```python
from build123d import *

# Parameters (mm, degrees)
F1_DEPTH = 12.7


with BuildPart() as f1:
    # F0 (on Top) → F1 (new body)
    with BuildSketch(Plane.XY):
        Polygon((-6.950833, -2.485712), (-10.236463, 1.818153), (-14.623778, -1.531184), (-11.338149, -5.835049), align=None)
        Polygon((-14.623778, -1.531184), (-10.236463, 1.818153), (-9.502501, 7.288792), (-12.851838, 11.676108), (-18.322477, 12.410069), (-22.709792, 9.060732), (-23.443754, 3.590093), (-20.094417, -0.797222), align=None)
    extrude(amount=F1_DEPTH)


solid = f1.part
```
Can you work these out from the model? Positions are in its coordinate system, mm. A direction names the side the tool comes from. Coordinates: 2 decimals unless noted, no trailing zeros. Loops run counter-clockwise (first coordinate to the right, second up) from the corner with the lowest first, then second, coordinate; pieces in that order, holes last. Notation, with made-up numbers: (-20.75, 57.25) -> (37.25, 57.25) arc R11 ccw to (37.25, 65.25) -> close; hole circle Ø11 at (-2.75, 18). An arc over 180 degrees is marked (long way). Put each result on its own line as item: value. Start each with the question number.
Q1. I'm going to push flat-ended pins straight in: P1, Ø5, axis at x = -14.5, z = 5.5, coming from the +Y side; P2, Ø4, axis at y = -2.5, z = 2.5, coming from the -X side; P3, Ø1, axis at x = -12, y = -2.5, coming from the -Z side. Where does each tip first touch, or does it pass through?
Q2. If I drill on line 1 (Y direction, x = -20.75, z = 2.25); line 2 (Y direction, x = -13.5, z = 8.25); line 3 (X direction, y = 1.5, z = 9), over which ranges is the centre line in solid material (lowest first)? Write a range as [from, to].
Q3. For faces 1 (the face through (-9.875, 4.515, 6.261)), 2 (the face through (-21.793, 1.427, 6.261)), which set-ups out of +Z, -Z, +X, -X, +Y, -Y let a thin tool reach every point of the face, with its end or its side?
Q4. Thinking about a two-plate mould opening in Y: for faces 3 (the face through (-17.4, -1.16, 6.26)), 4 (the face through (-8.571, -0.364, 6.261)), 5 (the face through (-15, 3, 0)), which applies, pulls with the +Y half, pulls with the -Y half, needs draft (parallel to the pull), parting line crosses it, or undercut?
Q5. I want a section at C-C (x = -19.75). Write out the boundary of the cut face in (y, z), plus the area to 3 significant figures.
Q6. I want a section at B-B (y = 5.5). Write out the boundary of the cut face in (x, z), plus the area to 3 significant figures.
Q7. I want a section at A-A (z = 8.75). Write out the boundary of the cut face in (x, y), plus the area to 3 significant figures.
Taken from the geometry:
1. P1: stops at y = 12.23
1. P2: stops at x = -20.32
1. P3: stops at z = 0
2. line 1: y = [0.06, 10.56]
2. line 2: y = [-3, 11.76]
2. line 3: x = [-21.85, -9.99]
3. face 1: +Z, -Z, +X
3. face 2: +Z, -Z, -X, -Y
4. face 3: pulls with the -Y half
4. face 4: undercut
4. face 5: needs draft
5. outline: (-0.84, 0) -> (11.32, 0) -> (11.32, 12.7) -> (-0.84, 12.7) -> close
5. area: 154 mm2
6. outline: (-23.19, 0) -> (-9.74, 0) -> (-9.74, 12.7) -> (-23.19, 12.7) -> close
6. area: 171 mm2
7. outline: (-23.44, 3.59) -> (-20.09, -0.8) -> (-14.62, -1.53) -> (-11.34, -5.84) -> (-6.95, -2.49) -> (-10.24, 1.82) -> (-9.5, 7.29) -> (-12.85, 11.68) -> (-18.32, 12.41) -> (-22.71, 9.06) -> close
7. area: 177 mm2
